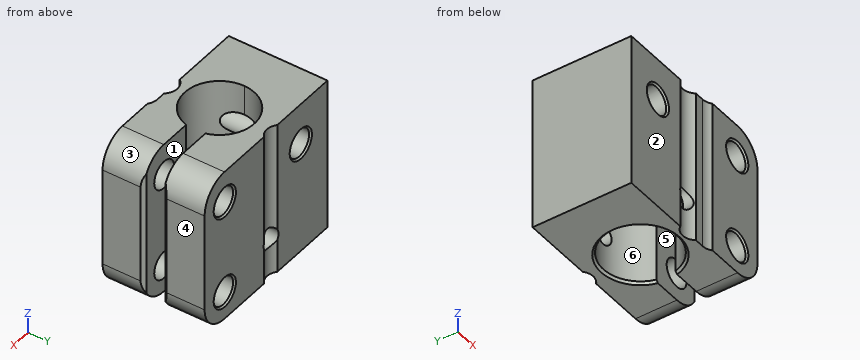
```python
from build123d import *

# Parameters (mm, degrees)
SKETCH1_W               = 39.2938
SKETCH1_H               = 35.2044
BOSS_EXTRUDE1_DEPTH     = 23.2664
CUT_EXTRUDE1_DEPTH      = 47.54756522
SKETCH3_R               = 8.4455
CUT_EXTRUDE2_DEPTH      = 18.669
SKETCH4_R               = 3.175
SKETCH4_R_2             = 2.38125
CUT_EXTRUDE3_DEPTH      = 36.173334977
CUT_EXTRUDE4_DEPTH      = 47.547565346
CUT_EXTRUDE5_DEPTH      = 47.547565346
FILLET1_R               = 6.35
CHAMFER1_SIZE           = 0.508
CHAMFER2_SIZE           = 0.381
CUT_EXTRUDE6_DEPTH      = 36.173335093
CUT_EXTRUDE6_DEPTH_BACK = 36.173335093


with BuildPart() as part:
    # Sketch1 → Boss-Extrude1 (new body)
    with BuildSketch(Plane(origin=(0, 0, 0), x_dir=(1, 0, 0), z_dir=(0, 1, 0))):
        Rectangle(SKETCH1_W, SKETCH1_H)
    extrude(amount=BOSS_EXTRUDE1_DEPTH)

    # Sketch2 → Cut-Extrude1 (cut, through all)
    with BuildSketch(Plane(origin=(0, 0, -17.6022), x_dir=(-1, 0, 0), z_dir=(0, 0, -1))):
        with BuildLine():
            Line((-6.477, 11.6332), (-19.6469, 11.6332))
            Line((-19.6469, 11.6332), (-19.6469, 9.4361))
            Line((-19.6469, 9.4361), (-6.166862443, 9.4361))
            ThreePointArc((-6.166862443, 9.4361), (-6.399083184, 10.523759407), (-6.477, 11.6332))
        make_face()
        with BuildLine():
            Line((-19.6469, 13.8303), (-19.6469, 11.6332))
            Line((-19.6469, 11.6332), (-6.477, 11.6332))
            ThreePointArc((-6.477, 11.6332), (-6.399083184, 12.742640593), (-6.166862443, 13.8303))
            Line((-6.166862443, 13.8303), (-19.6469, 13.8303))
        make_face()
        with BuildLine():
            ThreePointArc((-6.166862443, 13.8303), (-6.399083184, 12.742640593), (-6.477, 11.6332))
            Line((-6.477, 11.6332), (9.398, 11.6332))
            ThreePointArc((9.398, 11.6332), (2.569940593, 19.492783184), (-6.166862443, 13.8303))
        make_face()
        with BuildLine():
            Line((9.398, 11.6332), (-6.477, 11.6332))
            ThreePointArc((-6.477, 11.6332), (-6.399083184, 10.523759407), (-6.166862443, 9.4361))
            ThreePointArc((-6.166862443, 9.4361), (2.569940593, 3.773616816), (9.398, 11.6332))
        make_face()
    extrude(amount=-CUT_EXTRUDE1_DEPTH, mode=Mode.SUBTRACT)

    # Sketch3 → Cut-Extrude2 (cut)
    with BuildSketch(Plane(origin=(0, 0, -17.6022), x_dir=(-1, 0, 0), z_dir=(0, 0, -1))):
        with Locations((1.4605, 11.6332)):
            Circle(SKETCH3_R)
    extrude(amount=-CUT_EXTRUDE2_DEPTH, mode=Mode.SUBTRACT)

    # Sketch4 → Cut-Extrude3 (cut, through all)
    with BuildSketch(Plane.XZ):
        with Locations(Location((13.189602751, -11.2522, 0), (0, 0, 270))):
            Circle(SKETCH4_R)
        with Locations(Location((13.189602751, 10.3378, 0), (0, 0, 270))):
            Circle(SKETCH4_R)
        with Locations(Location((-1.605897249, -8.7122, 0), (0, 0, 270))):
            Circle(SKETCH4_R_2)
        with Locations(Location((-11.130897249, 8.0518, 0), (0, 0, 270))):
            Circle(SKETCH4_R)
    extrude(amount=-CUT_EXTRUDE3_DEPTH, mode=Mode.SUBTRACT)

    # Sketch5 → Cut-Extrude4 (cut, through all)
    with BuildSketch(Plane(origin=(0, 0, -17.6022), x_dir=(-1, 0, 0), z_dir=(0, 0, -1))):
        with BuildLine():
            Line((-0.688916377, 23.2664), (3.609916377, 23.2664))
            ThreePointArc((3.609916377, 23.2664), (1.4605, 22.4282), (-0.688916377, 23.2664))
        make_face()
    extrude(amount=-CUT_EXTRUDE4_DEPTH, mode=Mode.SUBTRACT)

    # Sketch7 → Cut-Extrude5 (cut, through all)
    with BuildSketch(Plane(origin=(0, 0, -17.6022), x_dir=(-1, 0, 0), z_dir=(0, 0, -1))):
        with BuildLine():
            Line((-1.043201365, 0.762), (3.964201365, 0.762))
            ThreePointArc((3.964201365, 0.762), (1.4605, 1.984538867), (-1.043201365, 0.762))
        make_face()
        with BuildLine():
            Line((19.6469, 0), (19.6469, 0.762))
            Line((19.6469, 0.762), (3.964201365, 0.762))
            Line((3.964201365, 0.762), (-1.043201365, 0.762))
            Line((-1.043201365, 0.762), (-3.2131, 0.762))
            ThreePointArc((-3.2131, 0.762), (-4.312952263, 0.565414007), (-5.276605755, 0))
            Line((-5.276605755, 0), (19.6469, 0))
        make_face()
    extrude(amount=-CUT_EXTRUDE5_DEPTH, mode=Mode.SUBTRACT)

    # Fillet1
    fillet1_edges = [part.edges().sort_by_distance(p)[0] for p in [
        (19.6469, 4.71805, -17.6022),
        (19.6469, 4.71805, 17.6022),
        (19.6469, 18.54835, -17.6022),
        (19.6469, 18.54835, 17.6022),
    ]]
    fillet(fillet1_edges, radius=FILLET1_R)

    # Chamfer1
    chamfer1_edges = [part.edges().sort_by_distance(p)[0] for p in [
        (-9.906, 11.6332, -17.6022),
    ]]
    chamfer(chamfer1_edges, length=CHAMFER1_SIZE)

    # Chamfer2
    chamfer2_edges = [part.edges().sort_by_distance(p)[0] for p in [
        (-11.130897249, 0.762, 11.2268),
        (-11.130897249, 23.2664, 11.2268),
        (13.189602751, 23.2664, 13.5128),
        (13.189602751, 0, 13.5128),
        (13.189602751, 23.2664, -8.0772),
        (13.189602751, 0, -8.0772),
    ]]
    chamfer(chamfer2_edges, length=CHAMFER2_SIZE)

    # Sketch8 → Cut-Extrude6 (cut, two sides: drawn at the far end of the back side and taken through both)
    with BuildSketch(Plane.XY.offset(-CUT_EXTRUDE6_DEPTH_BACK)):
        Polygon((18.8849, 13.8303), (19.6469, 14.5923), (19.6469, 13.8303), align=None)
        Polygon((18.8849, 9.4361), (19.6469, 8.6741), (19.6469, 9.4361), align=None)
    extrude(amount=CUT_EXTRUDE6_DEPTH + CUT_EXTRUDE6_DEPTH_BACK, mode=Mode.SUBTRACT)


solid = part.part
```
Source: CAD feature listing. Evaluate the final solid. Frame: model axes, mm. Face numbers are marked on the shaded views. A direction names the side the tool comes from. Round coordinates to 2 decimals unless told otherwise and drop trailing zeros.
(1) Contact query for flat-ended pins moving along their axis: pin 1 Ø6 at (x, z) = (-1.61, -8.71) entering from -Y; pin 2 Ø5 at (x, z) = (13, -12.5) entering from -Y; pin 3 Ø1.5 at (y, z) = (14.5, -13) entering from +X; pin 4 Ø4 at (x, y) = (3.5, 7) entering from -Z. Output: stop coordinate, or through.
From the geometry:
pin 1: stops at y = 0.76
pin 2: stops at y = 0
pin 3: stops at x = 19.57
pin 4: stops at z = -17.44
(2) Pull-direction query (Y, two-part tool) for the marked faces 1, 2 and 3; classes: +Y half, -Y half, draft (parallel to the pull), parting line (faces both ways), or undercut.
From the geometry:
face 1: undercut
face 2: -Y half
face 3: draft
(3) Access query for the marked faces 4, 5 and 6. Directions: +Z, -Z, +X, -X, +Y, -Y. A direction counts if a zero-diameter tool reaches every point of the face in a straight line with its end or side. Return the directions, or none.
From the geometry:
face 4: +Z, -Z, +X, +Y, -Y
face 5: +Z, -Z, +X
face 6: -Z
(4) Section query B-B (y = 16.5). Give the number of separate pieces and of enclosed holes in the cut face, and give its area (3 significant figures).
From the geometry:
separate pieces: 2
enclosed holes: 3
area: 806 mm2
(5) Material intervals for probe 1 along Y at (x, z) = (17, -9); probe 2 along X at (y, z) = (5, 10.5); probe 3 along Y at (x, z) = (6, -4) (3 decimals), sorted ascending.
From the geometry:
probe 1: y = 0 to 9.44, 13.83 to 23.27
probe 2: x = -19.65 to -13.15, -9.11 to -5.82, 2.9 to 10.02, 16.36 to 19.65
probe 3: y = 0 to 7.675, 15.591 to 23.266
